Input: part model. Units: mm. Frame: model coordinates. A direction names the side the tool comes from. Coordinates: 2 decimals unless noted, no trailing zeros. Write each loop counter-clockwise with the first axis right and the second up, starting at its lowest first coordinate (ties: lowest second). Pieces come first, ordered by that corner, then holes. Notation, with made-up numbers: (40, 28.5) -> (65, 28.5) arc R14 ccw to (65, 42.5) -> close; hole circle Ø8 at (-17, -31). An arc over 180 degrees is marked (long way). Use one line per item in the form item = value. Start each with the question number.
(1) Pull-direction query (X, two-part tool) for faces 1 (the face through (84.114, 17, 5)), 2 (the face through (36, 18, 0)), 3 (the face through (77.255, 42.464, 6.591)), 4 (the face through (-13.886, 17, 5)); classes: released by +X, released by -X, zero draft, split by the parting line, or undercut.
(2) Cut plane B-B on y = 37.5. Return the cut outline in (x, z).
(3) Set-up query: faces 5 (the face through (65.767, 18, 3)), 6 (the face through (-11.91, 29.26, 4.64)), 7 (the face through (21.355, -8.156, -1.972)). Return all of +Z, -Z, +X, -X, +Y, -Y with unobstructed straight access to the full face (end or side cutting, diameter ignored); none if empty.
(4) First-contact query: pin 1 (6 mm diameter, centred on x = 0, y = 17, fed in from +Z); pin 2 (2.5 mm diameter, centred on x = -9.89, y = -9.74, fed in from +Z); pin 3 (3.5 mm diameter, centred on x = 32.5, y = -5.5, fed in from +Z); pin 4 (3 mm diameter, centred on x = 68.5, y = 35.5, fed in from +Z). Flat tips, straight axial feed; report the tip coordinate or a pass-through.
(5) Cut plane A-A on z = 10.75. Return the cut outline in (x, y).
(6) Cut plane C-C on x = 41. Return the cut outline in (y, z), plus the area to 3 significant figures.
(7) Ray query, line 1 along X through (y, z) = (14, 2); line 2 along Y through (x, z) = (73, 1.5); line 3 along Y through (x, z) = (67.5, 2.5). Return the intervals inside material, ascending.
(8) Cut plane D-D on y = 28. Return the cut outline in (x, z).
```python
from build123d import *

# Parameters (mm, degrees)
ESQUISSE1_W             = 98
ESQUISSE1_H             = 63
ESQUISSE1_W_2           = 90
ESQUISSE1_H_2           = 55
BOSS_EXTRU_1_DEPTH      = 13
ESQUISSE2_W             = 98
ESQUISSE2_H             = 63
BOSS_EXTRU_2_DEPTH      = 4
ESQUISSE3_W             = 5
ESQUISSE3_H             = 31.5
BOSS_EXTRU_3_DEPTH      = 7
CONG_2_R                = 4
ESQUISSE6_R             = 4
BOSS_EXTRU_5_DEPTH      = 17
ESQUISSE7_R             = 1.5
ENL_V_MAT_EXTRU_2_DEPTH = 83.442016046
ESQUISSE8_R             = 3.5
ENL_V_MAT_EXTRU_3_DEPTH = 10
ESQUISSE9_R             = 3.5
ESQUISSE9_R_2           = 1.5
BOSS_EXTRU_6_DEPTH      = 3.5
ESQUISSE10_R            = 5
ENL_V_MAT_EXTRU_4_DEPTH = 4


with BuildPart() as part:
    # Esquisse1 → Boss.-Extru.1 (new body)
    with BuildSketch(Plane.XY):
        with Locations((35.11398795, 17.760869565)):
            Rectangle(ESQUISSE1_W, ESQUISSE1_H)
        with Locations((35.11398795, 17.760869565)):
            Rectangle(ESQUISSE1_W_2, ESQUISSE1_H_2, mode=Mode.SUBTRACT)
    extrude(amount=BOSS_EXTRU_1_DEPTH)

    # Esquisse2 → Boss.-Extru.2 (add)
    with BuildSketch(Plane(origin=(0, 0, 0), x_dir=(-1, 0, 0), z_dir=(0, 0, -1))):
        with Locations((-35.11398795, 17.760869565)):
            Rectangle(ESQUISSE2_W, ESQUISSE2_H)
    extrude(amount=BOSS_EXTRU_2_DEPTH)

    # Esquisse3 → Boss.-Extru.3 (add)
    with BuildSketch(Plane.XY):
        Polygon((80.11398795, 2.010869565), (80.11398795, 33.510869565), (80.11398795, 38.510869565), (65.766919995, 38.510869565), (65.766919995, 33.510869565), (65.766919995, 2.010869565), (65.766919995, -2.989130435), (80.11398795, -2.989130435), align=None)
        with Locations((73.11398795, 17.760869565)):
            Rectangle(ESQUISSE3_W, ESQUISSE3_H, mode=Mode.SUBTRACT)
    extrude(amount=BOSS_EXTRU_3_DEPTH)

    # Congé2
    cong_2_edges = [part.edges().sort_by_distance(p)[0] for p in [
        (-13.88601205, 49.260869565, 4.5),
        (84.11398795, 49.260869565, 4.5),
        (84.11398795, -13.739130435, 4.5),
        (-13.88601205, -13.739130435, 4.5),
    ]]
    fillet(cong_2_edges, radius=CONG_2_R)

    # Esquisse6 → Boss.-Extru.5 (add)
    with BuildSketch(Plane.XY.offset(13)):
        with Locations((-9.88601205, 45.260869565)):
            Circle(ESQUISSE6_R)
        with Locations((-9.88601205, -9.739130435)):
            Circle(ESQUISSE6_R)
        with Locations((80.11398795, -9.739130435)):
            Circle(ESQUISSE6_R)
        with Locations((80.11398795, 45.260869565)):
            Circle(ESQUISSE6_R)
    extrude(amount=-BOSS_EXTRU_5_DEPTH)

    # Esquisse7 → Enlèv. mat.-Extru.2 (cut)
    with BuildSketch(Plane.XY.offset(13)):
        with Locations((80.11398795, -9.739130435)):
            Circle(ESQUISSE7_R)
        with Locations((-9.88601205, -9.739130435)):
            Circle(ESQUISSE7_R)
        with Locations((-9.88601205, 45.260869565)):
            Circle(ESQUISSE7_R)
        with Locations((80.11398795, 45.260869565)):
            Circle(ESQUISSE7_R)
    extrude(amount=-ENL_V_MAT_EXTRU_2_DEPTH, mode=Mode.SUBTRACT)

    # Esquisse8 → Enlèv. mat.-Extru.3 (cut)
    with BuildSketch(Plane.XY):
        with Locations((22.11398795, -4.739130435)):
            Circle(ESQUISSE8_R)
        with Locations((40.11398795, -4.739130435)):
            Circle(ESQUISSE8_R)
    extrude(amount=-ENL_V_MAT_EXTRU_3_DEPTH, mode=Mode.SUBTRACT)

    # Esquisse9 → Boss.-Extru.6 (add)
    with BuildSketch(Plane.XY):
        with Locations((31.113164105, -4.617357959)):
            Circle(ESQUISSE9_R)
        with Locations((31.113164105, -4.617357959)):
            Circle(ESQUISSE9_R_2, mode=Mode.SUBTRACT)
    extrude(amount=BOSS_EXTRU_6_DEPTH)

    # Esquisse10 → Enlèv. mat.-Extru.4 (cut)
    with BuildSketch(Plane.ZY.offset(13.88601205)):
        with Locations(Location((4.424351408, 24.266648435, 0), (0, 0, 270))):
            Circle(ESQUISSE10_R)
    extrude(amount=-ENL_V_MAT_EXTRU_4_DEPTH, mode=Mode.SUBTRACT)


solid = part.part
```
Values:
q1.face_1 = released by +X
q1.face_2 = undercut
q1.face_3 = undercut
q1.face_4 = released by -X
q2.outline = (-13.89, -4) -> (84.11, -4) -> (84.11, 13) -> (80.11, 13) -> (80.11, 7) -> (65.77, 7) -> (65.77, 0) -> (-9.89, 0) -> (-9.89, 13) -> (-13.89, 13) -> close
q3.face_5 = +Z
q3.face_6 = -X
q3.face_7 = +Z, -Z
q4.pin_1 = 0
q4.pin_2 = through
q4.pin_3 = 3.5
q4.pin_4 = 7
q5.outline = (-13.89, -9.74) arc R4 ccw to (-9.89, -13.74) -> (80.11, -13.74) arc R4 ccw to (84.11, -9.74) -> (84.11, 45.26) arc R4 ccw to (80.11, 49.26) -> (-9.89, 49.26) arc R4 ccw to (-13.89, 45.26) -> close; hole circle Ø3 at (-9.89, -9.74); hole circle Ø3 at (-9.89, 45.26); hole (-9.89, -5.74) arc R4 cw to (-5.89, -9.74) -> (76.11, -9.74) arc R4 cw to (80.11, -5.74) -> (80.11, 41.26) arc R4 cw to (76.11, 45.26) -> (-5.89, 45.26) arc R4 cw to (-9.89, 41.26) -> close; hole circle Ø3 at (80.11, -9.74); hole circle Ø3 at (80.11, 45.26)
q6.outline = (-13.74, -4) -> (-8.13, -4) -> (-8.13, 0) -> (-9.74, 0) -> (-9.74, 13) -> (-13.74, 13) -> close; (-1.35, -4) -> (49.26, -4) -> (49.26, 13) -> (45.26, 13) -> (45.26, 0) -> (-1.35, 0) -> close
q6.area = 329 mm2
q7.line_1 = -13.89 to -9.89, 65.77 to 70.61, 75.61 to 84.11
q7.line_2 = -13.74 to -9.74, -2.99 to 2.01, 33.51 to 38.51, 45.26 to 49.26
q7.line_3 = -13.74 to -9.74, -2.99 to 38.51, 45.26 to 49.26
q8.outline = (-13.89, -4) -> (84.11, -4) -> (84.11, 13) -> (80.11, 13) -> (80.11, 7) -> (75.61, 7) -> (75.61, 0) -> (70.61, 0) -> (70.61, 7) -> (65.77, 7) -> (65.77, 0) -> (-9.89, 0) -> (-9.89, 1.1) -> (-13.89, 1.1) -> close; (-13.89, 7.75) -> (-9.89, 7.75) -> (-9.89, 13) -> (-13.89, 13) -> close
